Verification items for the finished model (mm, model axes). A direction names the side the tool comes from. Give positions to 0.01 mm unless a question says otherwise; leave off trailing zeros. Loops run counter-clockwise (first coordinate to the right, second up) from the corner with the lowest first, then second, coordinate; pieces in that order, holes last. Notation, with made-up numbers: (21.5, 54) - (75.5, 54) arc R24 cw to (75.5, 68) - close; hole circle Ø3 at (24, -34.75). An arc over 180 degrees is marked (long way). One line per question, with ' | ' between items. Start each with the question number.
1. Section check A-A, the plane z = 0. Enter the section's corners in (x, y).
2. Thickness scan on line 1 along Z through (x, y) = (0, 5.75); line 2 along X through (y, z) = (3.75, -1.75). Record the ranges inside material, lowest first. Write a range as from..to.
3. Tool access check on faces 1 (the face through (-2.065, 1.109, -1.253)), 2 (the face through (2.86, 4.93, 0.9)). Record the directions out of +Z, -Z, +X, -X, +Y, -Y that give a thin tool (end or side, any length) a straight path to the whole face; none if there is none.
4. Mould release check, pull along Y, two halves, no side actions. Record for faces 3 (the face through (-2.27, 4.25, -0.04)), 4 (the face through (1, 10, -2)), 5 (the face through (-2.065, 1.141, 1.246)): +Y half, -Y half, draft (parallel to the pull), parting line (faces both ways), or undercut.
5. Depth check by flat-ended pin: pin 1 Ø1.5 at (y, z) = (3, 0) entering from -X; pin 2 Ø1.5 at (y, z) = (4.5, -2) entering from -X. Enter the tip coordinate at first touch or a pass-through.
6. Section check D-D, the plane x = -2.25. Enter the section's corners in (y, z), then the cut area to 3 significant figures.
7. Section check C-C, the plane y = 6.25. Enter the section's corners in (x, z).
8. Section check B-B, the plane x = 0. Enter the section's corners in (y, z).
from build123d import *

# Parameters (mm, degrees)
F0_R     = 3
F1_DEPTH = 10
F3_DEPTH = 25
F4_R     = 2
F5_DEPTH = 25


with BuildPart() as f1:
    # F0 (on Front) → F1 (new body)
    with BuildSketch(Plane.XZ):
        Circle(F0_R)
    extrude(amount=-F1_DEPTH)

    # F2 (on Right) → F3 (cut)
    with BuildSketch(Plane.YZ):
        with BuildLine():
            Line((0, 1.5), (0, 0))
            Line((0, 0), (0, -1.5))
            Line((0, -1.5), (2.25, -1))
            ThreePointArc((2.25, -1), (4.25, 0), (2.25, 1))
            Line((2.25, 1), (0, 1.5))
        make_face()
    extrude(amount=-F3_DEPTH, mode=Mode.SUBTRACT)

    # F4 (on Front) → F5 (cut)
    with BuildSketch(Plane.XZ):
        Circle(F4_R)
    extrude(amount=-F5_DEPTH, mode=Mode.SUBTRACT)


solid = f1.part
Results list:
1) outline: (-3, 4.25) - (-2, 4.25) - (-2, 10) - (-3, 10) - close; (2, 0) - (3, 0) - (3, 10) - (2, 10) - close
2) line 1: -3..-2, 2..3 | line 2: -2.44..-0.97, 0.97..2.44
3) face 1: -X, -Y | face 2: +Y, -Y
4) face 3: undercut | face 4: +Y half | face 5: -Y half
5) pin 1: x = 1.85 | pin 2: x = -2.73
6) outline: (0, -1.98) - (10, -1.98) - (10, 1.98) - (0, 1.98) - (0, 1.5) - (2.25, 1) arc R1.25 cw (long way) to (2.25, -1) - (0, -1.5) - close | area: 29.9 mm²
7) outline: circle Ø6 at (0, 0); hole circle Ø4 at (0, 0)
8) outline: (0, -3) - (10, -3) - (10, -2) - (0, -2) - close; (0, 2) - (10, 2) - (10, 3) - (0, 3) - close
